from build123d import *

# Parameters (mm, degrees)
BOX001_W        = 24
BOX001_H        = 14
BOX001_DEPTH    = 11.5
SKETCH001_R     = 4.2
POCKET001_DEPTH = 14
SKETCH002_R     = 1.5
POCKET002_DEPTH = 11.501
FILLET003_R     = 3


with BuildPart() as part:
    # Box001 → Box001 (new body)
    with BuildSketch(Plane(origin=(-2.5, 17, 0), x_dir=(1, 0, 0), z_dir=(0, 0, 1))):
        with Locations((12, 7)):
            Rectangle(BOX001_W, BOX001_H)
    extrude(amount=BOX001_DEPTH)

    # Sketch001 → Pocket001 (cut)
    with BuildSketch(Plane(origin=(-2.5, 31, 0), x_dir=(-1, 0, 0), z_dir=(0, 1, 0))):
        with Locations((-12, 11.35)):
            Circle(SKETCH001_R)
    extrude(amount=-POCKET001_DEPTH, mode=Mode.SUBTRACT)

    # Sketch002 → Pocket002 (cut, through all)
    with BuildSketch(Plane(origin=(-2.5, 17, 0), x_dir=(1, 0, 0), z_dir=(0, 0, -1))):
        with Locations((4, -7)):
            Circle(SKETCH002_R)
        with Locations((20, -7)):
            Circle(SKETCH002_R)
    extrude(amount=-POCKET002_DEPTH, mode=Mode.SUBTRACT)

    # Fillet003
    fillet003_edges = [part.edges().sort_by_distance(p)[0] for p in [
        (-2.5, 31, 5.75),
        (21.5, 31, 5.75),
    ]]
    fillet(fillet003_edges, radius=FILLET003_R)


solid = part.part
Source: CAD feature listing. Evaluate the final solid. Frame: model axes, mm. Round coordinates to 2 decimals unless told otherwise and drop trailing zeros. Loops run counter-clockwise (first coordinate to the right, second up) from the corner with the lowest first, then second, coordinate; pieces in that order, holes last. Notation, with made-up numbers: (39.25, -35) -> (67.25, -35) arc R34 cw to (67.25, 1) -> close; hole circle Ø10 at (-6.5, 73.25). An arc over 180 degrees is marked (long way). Answer as a JSON object with one key per item and string values. Group by question number.
Q1. Mould query, pull axis Y, two halves, no side actions, for faces 1 (the flat face through (21.5, 22, 6)), 2 (the flat face through (9, 31, 4)), 3 (the cylindrical face through (16.39, 22.99, 5.67)). Classes: pulls with the +Y half, pulls with the -Y half, needs draft (parallel to the pull), parting line crosses it, or undercut.
Q2. Section query B-B (y = 24). Output: boundary loops of the cut face in (x, z), plus the area to 3 significant figures.
Q3. Section query C-C (z = 7.5). Output: boundary loops of the cut face in (x, y), plus the area to 3 significant figures.
Q4. Section query A-A (x = 17.5). Output: boundary loops of the cut face in (y, z), plus the area to 4 significant figures.
Q5. Section query D-D (z = 4.75). Output: boundary loops of the cut face in (x, y), plus the area to 3 significant figures.
Q6. Contact query for a flat-ended pin moving along its axis: P1, Ø1.8, axis at x = 1.5, y = 24, coming from the -Z side. Output: stop coordinate, or through.
Q7. Ray query, line 1 (X direction, y = 24, z = 5.25); line 2 (X direction, y = 24, z = 8.75); line 3 (Y direction, x = 1.5, z = 5.75). Return the intervals inside material, ascending. Write a range as from..to.
Completed:
{
 "1": {"face 1": "needs draft", "face 2": "pulls with the +Y half", "face 3": "undercut"},
 "2": {"outline": "(-2.5, 0) -> (0, 0) -> (0, 11.5) -> (-2.5, 11.5) -> close; (3, 0) -> (16, 0) -> (16, 11.5) -> (13.7, 11.5) arc R4.2 cw (long way) to (5.3, 11.5) -> (3, 11.5) -> close; (19, 0) -> (21.5, 0) -> (21.5, 11.5) -> (19, 11.5) -> close", "area": "178 mm²"},
 "3": {"outline": "(-2.5, 17) -> (7.82, 17) -> (7.82, 31) -> (0.5, 31) arc R3 ccw to (-2.5, 28) -> close; (11.18, 17) -> (21.5, 17) -> (21.5, 28) arc R3 ccw to (18.5, 31) -> (11.18, 31) -> close; hole circle Ø3 at (1.5, 24); hole circle Ø3 at (17.5, 24)", "area": "271 mm²"},
 "4": {"outline": "(17, 0) -> (22.5, 0) -> (22.5, 11.5) -> (17, 11.5) -> close; (25.5, 0) -> (31, 0) -> (31, 11.5) -> (25.5, 11.5) -> close", "area": "126.5 mm²"},
 "5": {"outline": "(-2.5, 17) -> (21.5, 17) -> (21.5, 28) arc R3 ccw to (18.5, 31) -> (0.5, 31) arc R3 ccw to (-2.5, 28) -> close; hole circle Ø3 at (1.5, 24); hole circle Ø3 at (17.5, 24)", "area": "318 mm²"},
 "6": {"P1": "through"},
 "7": {"line 1": "-2.5..0, 3..16, 19..21.5", "line 2": "-2.5..0, 3..6.2, 12.8..16, 19..21.5", "line 3": "17..22.5, 25.5..31"}
}
